Autodesk Inventor part; units mm, degrees
ref_plane "YZ Plane" through (0, 0, 0) normal (1, 0, 0) x (0, 1, 0)
ref_plane "XZ Plane" through (0, 0, 0) normal (0, 1, 0) x (-1, 0, 0)
ref_plane "XY Plane" through (0, 0, 0) normal (0, 0, 1) x (1, 0, 0)
sketch "Sketch1" plane through (0, 0, 0) normal (0, 0, 1) x (1, 0, 0)
  circle A0 centre (0, 0) radius 30
  circle A1 centre (0, 0) radius 32
  dimension "d0" = 60
  dimension "d1" = 2
extrude "Extrusion1" add sketch "Sketch1" along normal blind 100
sketch "Sketch2" plane through (0, 0, 100) normal (0, 0, 1) x (1, 0, 0)
  circle A0 centre (0, 0) radius 34
  circle A1 centre (0, 0) radius 32
  circle A2 centre (0, 0) radius 30
  dimension "d4" = 2
extrude "Extrusion2" add sketch "Sketch2" along normal blind 2 contours A0 | A1
sketch "Sketch3" plane through (0, 0, 102) normal (0, 0, 1) x (1, 0, 0)
  circle A0 centre (0, 0) radius 3.25
  arc A1 (-4.5086, 5.6776) -> (4.5086, 5.6776) centre (0, 0) ccw
  line L0 (-4.5086, 5.6776) -> (-4.5086, 29.6593)
  circle A2 centre (0, 0) radius 30
  line L1 (4.5086, 5.6776) -> (4.5086, 29.6593)
  dimension "d7" = 6.5
  dimension "d8" = 4
extrude "Extrusion3" add sketch "Sketch3" against normal blind 4 contours L0 A2 L1 A1 picked at (0.5026, 13.7724)
pattern_circular "Circular Pattern1" count 3 over 360 about axis through (0, 0, 0) along (0, 0, 1) of "Extrusion3"
properties part number "Bobbin-Emma"
Source: CAD feature listing. Evaluate the final solid. Frame: model axes, mm. A direction names the side the tool comes from. Give positions to 0.01 mm unless a question says otherwise; leave off trailing zeros. Order: outer loops, then holes, each group sorted by start corner. A loop starts at its lowest first (then second) coordinate and runs counter-clockwise, first axis right, second up.
(1) Section query B-B (y = -9.5). Return the cut outline in (x, z).
(2) Material intervals for line 1 along Y through (x, z) = (0, 99.7); line 2 along Y through (x, z) = (0, 100.5); line 3 along Y through (x, z) = (0, 23), sorted ascending.
(3) Section query A-A (x = 0). Return the cut outline in (y, z), plus the area to 3 significant figures.
(4) Access query for faces 1 (the face through (2, 4, 98)), 2 (the face through (-5.89, 3.95, 102)), 3 (the face through (12.902, -12.655, 100.028)). Directions: +Z, -Z, +X, -X, +Y, -Y. A direction counts if a zero-diameter tool reaches every point of the face in a straight line with its end or side. Return the directions, or none.
(5) Pull-direction query (Y, two-part tool) for faces 4 (the face through (-6.94, 31.24, 49.3)), 5 (the face through (-23, -23, 100)), 6 (the face through (-6.26, 3.66, 100.03)), 7 (the face through (4.509, 18, 100)); classes: +Y half, -Y half, draft (parallel to the pull), parting line (faces both ways), or undercut.
(6) Section query C-C (x = 25.5). Return the cut outline in (y, z).
(7) Section query D-D (y = -20). Return the cut outline in (x, z), plus the area to 3 significant figures.
(8) Contact query for flat-ended pins moving along their axis: P1, Ø6, axis at x = -1.5, y = -1.5, coming from the +Z side; P2, Ø12, axis at x = -16, z = 48.5, coming from the -Y side; P3, Ø4.5, axis at y = 14, z = 99, coming from the -X side; P4, Ø10, axis at x = 12.5, z = 87, coming from the +Y side. Output: stop coordinate, or through.
Outcome:
1. outline: (-32.65, 100) - (-30.56, 100) - (-30.56, 0) - (-28.46, 0) - (-28.46, 102) - (-32.65, 102) - close; (-25.47, 98) - (-7.44, 98) - (-7.44, 102) - (-25.47, 102) - close; (7.44, 98) - (25.47, 98) - (25.47, 102) - (7.44, 102) - close; (28.46, 0) - (30.56, 0) - (30.56, 100) - (32.65, 100) - (32.65, 102) - (28.46, 102) - close
2. line 1: y = -32 to -30, -7.25 to -3.25, 3.25 to 32
2. line 2: y = -34 to -30, -7.25 to -3.25, 3.25 to 34
2. line 3: y = -32 to -30, 30 to 32
3. outline: (-34, 100) - (-32, 100) - (-32, 0) - (-30, 0) - (-30, 102) - (-34, 102) - close; (-7.25, 98) - (-3.25, 98) - (-3.25, 102) - (-7.25, 102) - close; (3.25, 98) - (30, 98) - (30, 0) - (32, 0) - (32, 100) - (34, 100) - (34, 102) - (3.25, 102) - close
3. area: 539 mm2
4. face 1: -Z
4. face 2: +Z, +X, -X, +Y, -Y
4. face 3: +Z, -Z
5. face 4: parting line
5. face 5: draft
5. face 6: undercut
5. face 7: undercut
6. outline: (-22.49, 100) - (-19.33, 100) - (-19.33, 0) - (-15.8, 0) - (-15.8, 98) - (-9.52, 98) - (-9.52, 102) - (-22.49, 102) - close; (15.8, 0) - (19.33, 0) - (19.33, 100) - (22.49, 100) - (22.49, 102) - (15.8, 102) - close
7. outline: (-27.5, 100) - (-24.98, 100) - (-24.98, 0) - (-22.36, 0) - (-22.36, 102) - (-27.5, 102) - close; (22.36, 0) - (24.98, 0) - (24.98, 100) - (27.5, 100) - (27.5, 102) - (22.36, 102) - close
7. area: 544 mm2
8. P1: stops at z = 102
8. P2: stops at y = -30.4
8. P3: stops at x = -31.82
8. P4: stops at y = 31.11
